Build history of the part. All positions in model axes, mm. A direction names the side the tool comes from. Give positions to 0.01 mm unless a question says otherwise; leave off trailing zeros. Order: outer loops, then holes, each group sorted by start corner. A loop starts at its lowest first (then second) coordinate and runs counter-clockwise, first axis right, second up. Notation, with made-up numbers: (-22.5, -16) -> (-4.5, -16) arc R29 cw to (-4.5, 9) -> close; hole circle Ø11 at (75, 37.5). An arc over 180 degrees is marked (long way). One line per question, with ' | ' between items. Start each with the question number.
(1) Cut at C-C (y = -26). Give the cut face in (x, z).
(2) Pin check, flat tips, straight feed: pin 1 Ø5 at (x, y) = (-61.5, -17) entering from +Z; pin 2 Ø0.6 at (x, y) = (-45.5, -3.5) entering from +Z. Stop position of each tip, or through.
(3) Cut at B-B (x = -67.5). Give the cut face in (y, z), then the cut area to 3 significant figures.
(4) Pull direction Y, two halves, no side cores. Call faces 1 (the face through (-44, -0.219, 13)), 2 (the face through (-44, -6.569, 16)), 3 (the face through (-0.76, -3.4, 26.65)): +Y half, -Y half, draft (parallel to the pull), parting line (faces both ways), or undercut.
(5) Which spindle directions (+Z, -Z, +X, -X, +Y, -Y) get a long thin tool onto all of the face, cutting with end or side? Do faces 4 (the face through (-88.14, -22.7, 6.33)), 5 (the face through (-0.76, -5.84, 14.54)), 6 (the face through (-46.32, -5.81, 26.65)), 7 (the face through (-0.764, -0.944, 12.942)). Say none if no direction does.
(6) Drill centre lines: L1, parallel to Y at x = -41, z = 10; L2, parallel to Z at x = -11.5, y = -23; L3, parallel to Y at x = -20.5, z = 38. Where is each one in solid material? Low to high. Write a range as from..to.
(7) Cut at D-D (z = 31). Give the cut face in (x, y).
(8) Cut at A-A (z = 12.5). Give the cut face in (x, y).
from build123d import *

# Parameters (mm, degrees)
F1_DEPTH = 88.9
F2_R     = 2.54


with BuildPart() as f1:
    # F0 (on Right) → F1 (new body)
    with BuildSketch(Plane.YZ):
        Polygon((-38.319263, 51.508548), (-44.669263, 51.508548), (-44.669263, 0.708548), (-0.219263, 0.708548), (-0.219263, 27.378548), (-6.569263, 27.378548), (-6.569263, 7.058548), (-38.319263, 7.058548), align=None)
    extrude(amount=-F1_DEPTH)

    # F2
    f2_edges = [f1.edges().sort_by_distance(p)[0] for p in [
        (-44.45, -0.219263, 27.378548),
        (-44.45, -6.569263, 27.378548),
        (-44.45, -38.319263, 51.508548),
        (-88.9, -6.569263, 17.218548),
        (-88.9, -22.444263, 7.058548),
        (-88.9, -38.319263, 29.283548),
        (-88.9, -44.669263, 26.108548),
        (-88.9, -41.494263, 51.508548),
        (-88.9, -0.219263, 14.043548),
        (0, -41.494263, 51.508548),
        (0, -38.319263, 29.283548),
        (0, -44.669263, 26.108548),
        (0, -22.444263, 7.058548),
        (0, -6.569263, 17.218548),
        (0, -3.394263, 27.378548),
        (0, -0.219263, 14.043548),
        (-44.45, -44.669263, 51.508548),
        (-44.45, -44.669263, 0.708548),
    ]]
    fillet(f2_edges, radius=F2_R)


solid = f1.part
Result set:
1) outline: (-88.9, 0.71) -> (0, 0.71) -> (0, 4.52) arc R2.54 ccw to (-2.54, 7.06) -> (-86.36, 7.06) arc R2.54 ccw to (-88.9, 4.52) -> close
2) pin 1: stops at z = 7.06 | pin 2: stops at z = 27.38
3) outline: (-44.67, 3.25) arc R2.54 ccw to (-42.13, 0.71) -> (-0.22, 0.71) -> (-0.22, 24.84) arc R2.54 ccw to (-2.76, 27.38) -> (-4.03, 27.38) arc R2.54 ccw to (-6.57, 24.84) -> (-6.57, 7.06) -> (-38.32, 7.06) -> (-38.32, 48.97) arc R2.54 ccw to (-40.86, 51.51) -> (-42.13, 51.51) arc R2.54 ccw to (-44.67, 48.97) -> close | area: 687 mm2
4) face 1: +Y half | face 2: undercut | face 3: draft
5) face 4: +Z, -X | face 5: +Z, +X | face 6: +Z, +X, -X | face 7: +Z, -Z, +X, +Y
6) L1: y = -44.67..-38.32, -6.57..-0.22 | L2: z = 0.71..7.06 | L3: y = -44.67..-38.32
7) outline: (-88.9, -42.13) arc R2.54 ccw to (-86.36, -44.67) -> (-2.54, -44.67) arc R2.54 ccw to (0, -42.13) -> (0, -40.86) arc R2.54 ccw to (-2.54, -38.32) -> (-86.36, -38.32) arc R2.54 ccw to (-88.9, -40.86) -> close
8) outline: (-88.9, -42.13) arc R2.54 ccw to (-86.36, -44.67) -> (-2.54, -44.67) arc R2.54 ccw to (0, -42.13) -> (0, -40.86) arc R2.54 ccw to (-2.54, -38.32) -> (-86.36, -38.32) arc R2.54 ccw to (-88.9, -40.86) -> close; (-88.9, -4.03) arc R2.54 ccw to (-86.36, -6.57) -> (-2.54, -6.57) arc R2.54 ccw to (0, -4.03) -> (0, -2.76) arc R2.54 ccw to (-2.54, -0.22) -> (-86.36, -0.22) arc R2.54 ccw to (-88.9, -2.76) -> close
